Can you work these out from the model? Positions are in its coordinate system, mm. A direction names the side the tool comes from. Coordinates: 2 decimals unless noted, no trailing zeros. Write each loop counter-clockwise with the first axis right and the second up, starting at its lowest first coordinate (ties: lowest second). Pieces come first, ordered by that corner, then holes. Notation, with made-up numbers: (71, 8) - (77, 8) arc R28 ccw to (77, 34) - close; hole circle Ø4 at (37.5, -12). An arc over 180 degrees is marked (long way). One line per question, with ' | ' between items. Start each with the question number.
from build123d import *

# Parameters (mm, degrees)
SKETCH_1_W          = 26
SKETCH_1_H          = 18
SKETCH_1_R          = 1.6
EXTRUDE_1_DEPTH     = 7.5
SKETCH_3_W          = 8
SKETCH_3_H          = 15
CUT_EXTRUDE_2_DEPTH = 30


with BuildPart() as part:
    # 草图1 → 凸台-拉伸1 (new, symmetric)
    with BuildSketch(Plane.XY):
        Rectangle(SKETCH_1_W, SKETCH_1_H)
        with Locations((-7.5, 0)):
            Circle(SKETCH_1_R, mode=Mode.SUBTRACT)
        with Locations(Location((7.5, 0, 0), (0, 0, 180))):
            Circle(SKETCH_1_R, mode=Mode.SUBTRACT)
    extrude(amount=EXTRUDE_1_DEPTH, both=True)

    # 草图3 → 切除-拉伸2 (cut)
    with BuildSketch(Plane.ZY.offset(13)):
        with Locations((0, 1.5)):
            Rectangle(SKETCH_3_W, SKETCH_3_H)
    extrude(amount=-CUT_EXTRUDE_2_DEPTH, mode=Mode.SUBTRACT)


solid = part.part
(1) Which directions (+Z, -Z, +X, -X, +Y, -Y) give clear straight access to the entire face, cutting with the end or side of a thin tool? Please do faces 5 (the face through (0, -6, 0)), 6 (the face through (0, 9, 6)).
(2) If we section it at C-C on x = -2: List the corners of the cut face in (y, z) for me, plus the area to 3 significant figures.
(3) I'm going to push flat-ended pins straight in: pin 1 (2.5 mm diameter, centred on x = -5, z = 0.5, fed in from +Y); pin 2 (5 mm diameter, centred on x = -7.5, y = 0, fed in from +Z). Where does each tip first touch, or does it pass through?
(4) If we mould it in two halves opening along Z, with no side actions, what happens to faces 1 (the face through (0, 0, -7.5)), 2 (the face through (0, 0, 7.5)), 3 (the face through (0, 9, -6)), 4 (the face through (0, 1, 4))? For each: +Z half, -Z half, draft (parallel to the pull), parting line (faces both ways), or undercut.
(5) If we section it at B-B on y = 2.5: List the corners of the cut face in (x, z) for me.
(6) If we section it at D-D on y = -1: List the corners of the cut face in (x, z) for me, plus the area to 3 significant figures.
(7) If we section it at A-A on x = 7.5: List the corners of the cut face in (y, z) for me, plus the area to 3 significant figures.
(8) If I drill on probe 1 along Z at (x, y) = (4.25, 3.25); probe 2 along Y at (x, z) = (-7.5, -6.5); probe 3 along X at (y, z) = (-0.25, 6.75), over which ranges is the centre line in solid material (lowest first)?
Values:
1) face 5: +X, -X, +Y | face 6: +Z, -Z, +X, -X, +Y
2) outline: (-9, -7.5) - (9, -7.5) - (9, -4) - (-6, -4) - (-6, 4) - (9, 4) - (9, 7.5) - (-9, 7.5) - close | area: 150 mm2
3) pin 1: y = -6 | pin 2: z = 7.5
4) face 1: -Z half | face 2: +Z half | face 3: draft | face 4: undercut
5) outline: (-13, -7.5) - (13, -7.5) - (13, -4) - (-13, -4) - close; (-13, 4) - (13, 4) - (13, 7.5) - (-13, 7.5) - close
6) outline: (-13, -7.5) - (-8.75, -7.5) - (-8.75, -4) - (-13, -4) - close; (-13, 4) - (-8.75, 4) - (-8.75, 7.5) - (-13, 7.5) - close; (-6.25, -7.5) - (6.25, -7.5) - (6.25, -4) - (-6.25, -4) - close; (-6.25, 4) - (6.25, 4) - (6.25, 7.5) - (-6.25, 7.5) - close; (8.75, -7.5) - (13, -7.5) - (13, -4) - (8.75, -4) - close; (8.75, 4) - (13, 4) - (13, 7.5) - (8.75, 7.5) - close | area: 147 mm2
7) outline: (-9, -7.5) - (-1.6, -7.5) - (-1.6, -4) - (-6, -4) - (-6, 4) - (-1.6, 4) - (-1.6, 7.5) - (-9, 7.5) - close; (1.6, -7.5) - (9, -7.5) - (9, -4) - (1.6, -4) - close; (1.6, 4) - (9, 4) - (9, 7.5) - (1.6, 7.5) - close | area: 128 mm2
8) probe 1: -7.5 to -4, 4 to 7.5 | probe 2: -9 to -1.6, 1.6 to 9 | probe 3: -13 to -9.08, -5.92 to 5.92, 9.08 to 13
